```python
from build123d import *

# Parameters (mm, degrees)
SKETCH2_W           = 44
SKETCH2_H           = 44
SKETCH2_R           = 2
SKETCH2_R_2         = 11.5
BOSS_EXTRUDE1_DEPTH = 5
SKETCH4_W           = 84
SKETCH4_H           = 34
SKETCH4_R           = 2.75
BOSS_EXTRUDE2_DEPTH = 7
BOSS_EXTRUDE3_DEPTH = 5
BOSS_EXTRUDE4_DEPTH = 5


with BuildPart() as part:
    # Sketch2 → Boss-Extrude1 (new body)
    with BuildSketch(Plane(origin=(0, 0, 0), x_dir=(1, 0, 0), z_dir=(0, 1, 0))):
        with Locations((22, 22)):
            Rectangle(SKETCH2_W, SKETCH2_H)
        with Locations((6.5, 37.5)):
            Circle(SKETCH2_R, mode=Mode.SUBTRACT)
        with Locations((6.5, 6.5)):
            Circle(SKETCH2_R, mode=Mode.SUBTRACT)
        with Locations((37.5, 6.5)):
            Circle(SKETCH2_R, mode=Mode.SUBTRACT)
        with Locations((37.5, 37.5)):
            Circle(SKETCH2_R, mode=Mode.SUBTRACT)
        with Locations((22, 22)):
            Circle(SKETCH2_R_2, mode=Mode.SUBTRACT)
    extrude(amount=BOSS_EXTRUDE1_DEPTH)

    # Sketch4 → Boss-Extrude2 (add)
    with BuildSketch(Plane(origin=(0, 0, -44), x_dir=(-1, 0, 0), z_dir=(0, 0, -1))):
        with Locations((-22, -12)):
            Rectangle(SKETCH4_W, SKETCH4_H)
        with Locations((-57, -19)):
            Circle(SKETCH4_R, mode=Mode.SUBTRACT)
        with Locations((13, -19)):
            Circle(SKETCH4_R, mode=Mode.SUBTRACT)
    extrude(amount=BOSS_EXTRUDE2_DEPTH)

    # Sketch5 → Boss-Extrude3 (add)
    with BuildSketch(Plane(origin=(44, 0, 0), x_dir=(0, 0, -1), z_dir=(1, 0, 0))):
        Polygon((0, 5), (51, 5), (51, -29), (44, -29), (0, 0), align=None)
    extrude(amount=BOSS_EXTRUDE3_DEPTH)

    # Sketch6 → Boss-Extrude4 (add)
    with BuildSketch(Plane.ZY):
        Polygon((-51, 5), (0, 5), (0, 0), (-44, -29), (-51, -29), align=None)
    extrude(amount=BOSS_EXTRUDE4_DEPTH)


solid = part.part
```
Here's how the part is built. I have some questions about the finished solid (model axes, mm). A direction names the side the tool comes from. Round coordinates to 2 decimals unless told otherwise and drop trailing zeros. Loops run counter-clockwise (first coordinate to the right, second up) from the corner with the lowest first, then second, coordinate; pieces in that order, holes last.
1. Suppose I cut it at D-D, the plane x = 57. Please give me the cut outline in (y, z), and give its area (4 significant figures).
Answers:
outline: (-29, -51) - (-21.75, -51) - (-21.75, -44) - (-29, -44) - close; (-16.25, -51) - (5, -51) - (5, -44) - (-16.25, -44) - close
area: 199.5 mm2
2. For faces 1 (the face through (-5, -8, -27)), 2 (the face through (0, -8, -31)), 3 (the face through (49, -8, -27)), 4 (the face through (46.5, -14.7, -22.3)), 5 (the face through (37.066, 2.465, -35.548)), which set-ups out of +Z, -Z, +X, -X, +Y, -Y let a thin tool reach every point of the face, with its end or its side?
Answers:
face 1: +Z, -X, +Y, -Y
face 2: +Z, -Y
face 3: +Z, +X, +Y, -Y
face 4: +Z, +X, -X, -Y
face 5: +Y, -Y
3. Suppose I cut it at B-B, the plane x = 37.5. Please give me the cut outline in (y, z).
Answers:
outline: (-29, -51) - (5, -51) - (5, -39.5) - (0, -39.5) - (0, -44) - (-29, -44) - close; (0, -35.5) - (5, -35.5) - (5, -8.5) - (0, -8.5) - close; (0, -4.5) - (5, -4.5) - (5, 0) - (0, 0) - close
4. If I drill on probe 1 along Z at (x, y) = (6.5, 2.55); probe 2 along Y at (x, z) = (-13, -45.75); probe 3 along X at (y, z) = (-4, -9), over which ranges is the centre line in solid material (lowest first)?
Answers:
probe 1: z = -51 to -39.5, -35.5 to -8.5, -4.5 to 0
probe 2: y = -29 to -21.75, -16.25 to 5
probe 3: x = -5 to 0, 44 to 49
5. Thinking about a two-plate mould opening in Z: for faces 6 (the face through (22, -14, -44)), 7 (the face through (21, 5, -36)), 8 (the face through (32.97, 2.46, -25.45)), 9 (the face through (36.026, 2.465, -7.852)), which applies, released by +Z, released by -Z, zero draft, split by the parting line, or undercut?
Answers:
face 6: released by +Z
face 7: zero draft
face 8: undercut
face 9: undercut
6. Suppose I cut it at C-C, the plane y = -18. Please give me the cut outline in (x, z).
Answers:
outline: (-20, -51) - (-15.56, -51) - (-15.56, -44) - (-20, -44) - close; (-10.44, -51) - (54.44, -51) - (54.44, -44) - (49, -44) - (49, -27.31) - (44, -27.31) - (44, -44) - (0, -44) - (0, -27.31) - (-5, -27.31) - (-5, -44) - (-10.44, -44) - close; (59.56, -51) - (64, -51) - (64, -44) - (59.56, -44) - close
7. Suppose I cut it at A-A, the plane z = -22. Please give me the cut outline in (x, y).
Answers:
outline: (-5, -14.5) - (0, -14.5) - (0, 0) - (10.5, 0) - (10.5, 5) - (-5, 5) - close; (33.5, 0) - (44, 0) - (44, -14.5) - (49, -14.5) - (49, 5) - (33.5, 5) - close
8. Will these pins go through, and if not, where does the flat tip stop? pin 1 (7 mm diameter, centred on x = -13, y = -19, fed in from -Z); pin 2 (17 mm diameter, centred on y = -16.5, z = -15, fed in from +X); pin 3 (16.5 mm diameter, centred on x = -13.5, y = -8.5, fed in from +Z); pin 4 (10 mm diameter, centred on y = -21, z = -35, fed in from -X).
Answers:
pin 1: stops at z = -51
pin 2: stops at x = 49
pin 3: stops at z = -44
pin 4: stops at x = -5
